For this review, use the dimensioned drawing (mm, ordinates from the lowest corner) and the shaded views. A direction names the side the tool comes from. Coordinates: 2 decimals unless noted, no trailing zeros. Loops run counter-clockwise (first coordinate to the right, second up) from the corner with the lowest first, then second, coordinate; pieces in that order, holes last. Notation, with made-up numbers: (15, 29) -> (69, 29) arc R26 cw to (69, 47) -> close; hole circle Ø9 at (29, -8.5). An arc over 180 degrees is marked (long way). Answer as a JSON object with one key per item and string values.
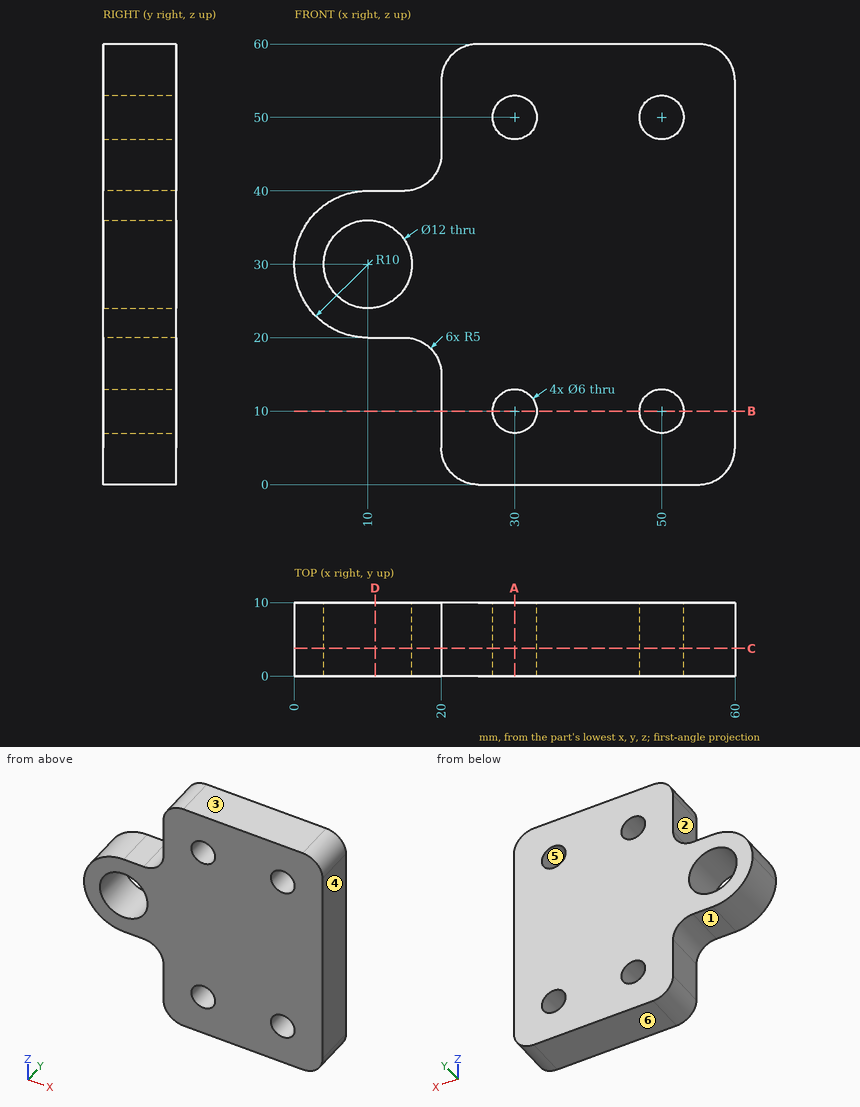
1) Wall thickness on probe 1 along Z at (x, y) = (30, 6.25); probe 2 along X at (y, z) = (4, 46.5); probe 3 along X at (y, z) = (6.75, 25.5): over which ranges is each line inside the solid? List them lowest first.
Completed:
{"probe 1": "0 to 7, 13 to 47, 53 to 60", "probe 2": "20 to 60", "probe 3": "1.07 to 6.03, 13.97 to 60"}
2) Clearance check with flat-ended pins moving along their axes: pin 1 Ø2.5 at (x, y) = (13.5, 7) entering from +Z; pin 2 Ø3 at (y, z) = (8.5, 9) entering from -X; pin 3 Ø4 at (x, y) = (12.5, 6) entering from -Z; pin 4 Ø5.5 at (x, z) = (30, 10) entering from +Y. State where each tip first meets the part, or that it passes through.
Completed:
{"pin 1": "z = 40", "pin 2": "x = 20", "pin 3": "z = 20", "pin 4": "through"}
3) For the marked faces 1, 2 and 3, list the 3-axis set-ups (+Z, -Z, +X, -X, +Y, -Y) from which the entire face can be reached by the end or side of a thin tool; tool diameter is ignored.
Completed:
{"face 1": "-Z, -X, +Y, -Y", "face 2": "+Z, -X, +Y, -Y", "face 3": "+Z, +X, -X, +Y, -Y"}
4) Add section D-D, the plane x = 11. Give the boundary of the cut face in (y, z).
Completed:
{"outline": "(0, 20) -> (10, 20) -> (10, 24.08) -> (0, 24.08) -> close; (0, 35.92) -> (10, 35.92) -> (10, 40) -> (0, 40) -> close"}
5) Add section C-C, the plane y = 3.75. Count the separate pieces of the cut face and the enclosed holes in it, and give its area (3 significant figures).
Completed:
{"separate pieces": "1", "enclosed holes": "5", "area": "2,520 mm²"}
6) The part is to be moulded in two halves that separate along Z. For the marked faces 4, 5 and 6, say which applies: pulls with the +Z half, pulls with the -Z half, needs draft (parallel to the pull), parting line crosses it, or undercut.
Completed:
{"face 4": "needs draft", "face 5": "undercut", "face 6": "pulls with the -Z half"}
7) Add section A-A, the plane x = 30. Give the boundary of the cut face in (y, z), and give its area (3 significant figures).
Completed:
{"outline": "(0, 0) -> (10, 0) -> (10, 7) -> (0, 7) -> close; (0, 13) -> (10, 13) -> (10, 47) -> (0, 47) -> close; (0, 53) -> (10, 53) -> (10, 60) -> (0, 60) -> close", "area": "480 mm²"}
8) Add section B-B, the plane z = 10. Give the boundary of the cut face in (x, y), and give its area (3 significant figures).
Completed:
{"outline": "(20, 0) -> (27, 0) -> (27, 10) -> (20, 10) -> close; (33, 0) -> (47, 0) -> (47, 10) -> (33, 10) -> close; (53, 0) -> (60, 0) -> (60, 10) -> (53, 10) -> close", "area": "280 mm²"}
